```python
from build123d import *

# Parameters (mm, degrees)
MODEL_R                 = 2
MODEL_R_2               = 1.5
MODEL_R_3               = 4.5
SALIENTE_EXTRUIR1_DEPTH = 3


with BuildPart() as part:
    # Model → Saliente-Extruir1 (new body)
    with BuildSketch(Plane.XY):
        with BuildLine():
            Line((206.945286968, 204.077019993), (199.609852846, 238.514519993))
            ThreePointArc((199.609852846, 238.514519993), (215.747807914, 258.452019993), (231.885762981, 238.514519993))
            Line((231.885762981, 238.514519993), (224.550328859, 204.077019993))
            ThreePointArc((224.550328859, 204.077019993), (215.747807914, 196.952019993), (206.945286968, 204.077019993))
        make_face()
        with Locations((215.747807914, 241.952019993)):
            Circle(MODEL_R, mode=Mode.SUBTRACT)
        with Locations((215.747807914, 232.952019993)):
            Circle(MODEL_R_2, mode=Mode.SUBTRACT)
        with Locations((215.747807914, 250.952019993)):
            Circle(MODEL_R_2, mode=Mode.SUBTRACT)
        with Locations((215.747807914, 205.952019993)):
            Circle(MODEL_R_3, mode=Mode.SUBTRACT)
        with BuildLine():
            Line((223.122807913, 245.202019993), (221.372807913, 245.202019993))
            ThreePointArc((221.372807913, 245.202019993), (220.842477828, 244.982350079), (220.622807913, 244.452019993))
            Line((220.622807913, 244.452019993), (220.622807913, 239.452019993))
            ThreePointArc((220.622807913, 239.452019993), (220.842477828, 238.921689907), (221.372807913, 238.702019993))
            Line((221.372807913, 238.702019993), (223.122807913, 238.702019993))
            ThreePointArc((223.122807913, 238.702019993), (223.653137999, 238.921689907), (223.872807913, 239.452019993))
            Line((223.872807913, 239.452019993), (223.872807913, 244.452019993))
            ThreePointArc((223.872807913, 244.452019993), (223.653137999, 244.982350079), (223.122807913, 245.202019993))
        make_face(mode=Mode.SUBTRACT)
        with BuildLine():
            Line((208.372807913, 245.202019993), (210.122807913, 245.202019993))
            ThreePointArc((210.122807913, 245.202019993), (210.653137999, 244.982350079), (210.872807913, 244.452019993))
            Line((210.872807913, 244.452019993), (210.872807913, 239.452019993))
            ThreePointArc((210.872807913, 239.452019993), (210.653137999, 238.921689907), (210.122807913, 238.702019993))
            Line((210.122807913, 238.702019993), (208.372807913, 238.702019993))
            ThreePointArc((208.372807913, 238.702019993), (207.842477828, 238.921689907), (207.622807913, 239.452019993))
            Line((207.622807913, 239.452019993), (207.622807913, 244.452019993))
            ThreePointArc((207.622807913, 244.452019993), (207.842477828, 244.982350079), (208.372807913, 245.202019993))
        make_face(mode=Mode.SUBTRACT)
    extrude(amount=SALIENTE_EXTRUIR1_DEPTH)


solid = part.part
```
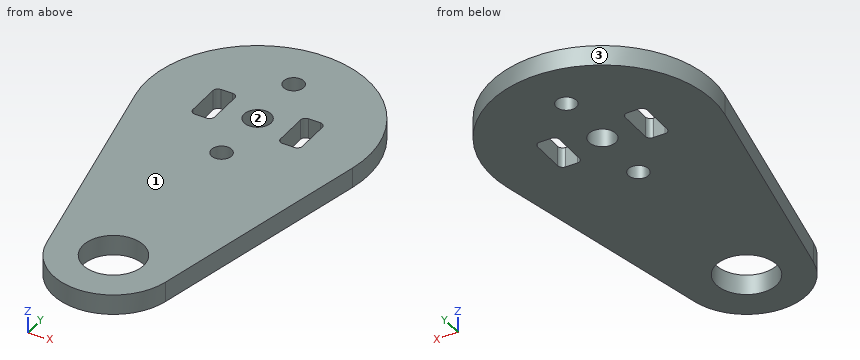
Input: part model. Units: mm. Frame: model coordinates. Face numbers are marked on the shaded views. Round coordinates to 2 decimals unless told otherwise and drop trailing zeros. Loops run counter-clockwise (first coordinate to the right, second up) from the corner with the lowest first, then second, coordinate; pieces in that order, holes last. Notation, with made-up numbers: (46.5, -34.5) -> (55.5, -34.5) arc R21 ccw to (55.5, -13.5) -> close; hole circle Ø2 at (-2, 36.5). An arc over 180 degrees is marked (long way). One line per item, written item: value.
(1) Section C-C (z = 2.15). Return the cut outline in (x, y).
Geometry check:
outline: (199.61, 238.51) -> (206.95, 204.08) arc R9 ccw to (224.55, 204.08) -> (231.89, 238.51) arc R16.5 ccw (long way) to start; hole (207.62, 239.45) arc R0.75 ccw to (208.37, 238.7) -> (210.12, 238.7) arc R0.75 ccw to (210.87, 239.45) -> (210.87, 244.45) arc R0.75 ccw to (210.12, 245.2) -> (208.37, 245.2) arc R0.75 ccw to (207.62, 244.45) -> close; hole circle Ø9 at (215.75, 205.95); hole circle Ø4 at (215.75, 241.95); hole circle Ø3 at (215.75, 232.95); hole circle Ø3 at (215.75, 250.95); hole (220.62, 239.45) arc R0.75 ccw to (221.37, 238.7) -> (223.12, 238.7) arc R0.75 ccw to (223.87, 239.45) -> (223.87, 244.45) arc R0.75 ccw to (223.12, 245.2) -> (221.37, 245.2) arc R0.75 ccw to (220.62, 244.45) -> close
(2) Material intervals for line 1 (Y direction, x = 218, z = 1.1); line 2 (Y direction, x = 214, z = 1.4); line 3 (Y direction, x = 217, z = 2.55), sorted ascending. Write a range as [from, to].
Geometry check:
line 1: [197.24, 202.06], [209.85, 258.3]
line 2: [197.12, 201.81], [210.1, 240.98], [242.92, 258.36]
line 3: [197.04, 201.63], [210.27, 232.13], [233.78, 240.39], [243.51, 250.13], [251.78, 258.4]
(3) Section B-B (y = 243). Return the cut outline in (x, z).
Geometry check:
outline: (199.28, 0) -> (207.62, 0) -> (207.62, 3) -> (199.28, 3) -> close; (210.87, 0) -> (214.04, 0) -> (214.04, 3) -> (210.87, 3) -> close; (217.45, 0) -> (220.62, 0) -> (220.62, 3) -> (217.45, 3) -> close; (223.87, 0) -> (232.21, 0) -> (232.21, 3) -> (223.87, 3) -> close
(4) Section A-A (y = 203). Return the cut outline in (x, z), plus the area to 3 significant figures.
Geometry check:
outline: (207.25, 0) -> (212.35, 0) -> (212.35, 3) -> (207.25, 3) -> close; (219.14, 0) -> (224.25, 0) -> (224.25, 3) -> (219.14, 3) -> close
area: 30.6 mm2
(5) Pin query (flat end, axial travel): pin 1 (4.5 mm diameter, centred on x = 215.75, y = 241.95, fed in from +Z); pin 2 (1 mm diameter, centred on y = 232, z = 1.5, fed in from -X); pin 3 (0.9 mm diameter, centred on x = 209, z = 2, fed in from -Y); pin 4 (1.5 mm diameter, centred on y = 226, z = 1.5, fed in from -X). Return the tip coordinate at first contact, or that it passes through.
Geometry check:
pin 1: z = 3
pin 2: x = 200.89
pin 3: y = 199.52
pin 4: x = 202.12
(6) Mould query, pull axis X, two halves, no side actions, for the marked faces 1, 2 and 3. Classes: pulls with the +X half, pulls with the -X half, needs draft (parallel to the pull), parting line crosses it, or undercut.
Geometry check:
face 1: needs draft
face 2: undercut
face 3: parting line crosses it
(7) Section D-D (x = 206). Return the cut outline in (y, z).
Geometry check:
outline: (208.51, 0) -> (255.26, 0) -> (255.26, 3) -> (208.51, 3) -> close
